Here's how the part is built. I have some questions about the finished solid (model axes, mm). A direction names the side the tool comes from. Round coordinates to 2 decimals unless told otherwise and drop trailing zeros. Write each loop counter-clockwise with the first axis right and the second up, starting at its lowest first coordinate (ties: lowest second). Pieces come first, ordered by that corner, then holes. Notation, with made-up numbers: (49, 35.5) -> (53, 35.5) arc R22 cw to (53, 56.5) -> close; hole circle Ø8 at (25.5, 5.25). An arc over 180 degrees is marked (long way). Answer in a Markdown table with one row per item.
from build123d import *

# Parameters (mm, degrees)
EXTRUDE_1_DEPTH                = 50
SPLIT_BODIES_1_SURFACE_1_BACK  = 226.829
SPLIT_BODIES_1_SURFACE_1_DEPTH = 453.658
SPLIT_BODIES_1_SURFACE_2_BACK  = 226.829
SPLIT_BODIES_1_SURFACE_2_DEPTH = 453.658


with BuildPart() as part:
    # 草图2 → 凸台-拉伸1 (new, symmetric)
    with BuildSketch(Plane.XY):
        with BuildLine():
            Line((120.381757685, 47.561632043), (136.603924057, 47.561632043))
            Line((136.603924057, 47.561632043), (146.850265064, 88.947420909))
            ThreePointArc((146.850265064, 88.947420909), (104.62030332, 85.070472378), (109.988846824, 127.136838271))
            Line((109.988846824, 127.136838271), (88.280849451, 128.197534042))
            ThreePointArc((88.280849451, 128.197534042), (80.571822415, 123.964886157), (80.863683371, 115.175163571))
            ThreePointArc((80.863683371, 115.175163571), (88.300101913, 100.587398022), (92.288223879, 84.706651578))
            Line((92.288223879, 84.706651578), (52.259104564, 84.706651578))
            Line((52.259104564, 84.706651578), (52.259104564, 37.347972633))
            Line((52.259104564, 37.347972633), (26.12059868, 28.530814049))
            Line((26.12059868, 28.530814049), (0, 28.530814049))
            Line((0, 28.530814049), (0, 0))
            Line((0, 0), (140.98, 0))
            Line((140.98, 0), (131.928221984, 26.834036233))
            Line((131.928221984, 26.834036233), (115.249995775, 26.834036233))
            Line((115.249995775, 26.834036233), (120.381757685, 47.561632043))
        make_face()
        with BuildLine():
            ThreePointArc((109.988846824, 127.136838271), (104.62030332, 85.070472378), (146.850265064, 88.947420909))
            Line((146.850265064, 88.947420909), (151.231226865, 106.642475172))
            ThreePointArc((151.231226865, 106.642475172), (147.884639105, 117.258207331), (140.564064785, 125.64287253))
            Line((140.564064785, 125.64287253), (109.988846824, 127.136838271))
        make_face()
        with BuildLine():
            ThreePointArc((140.564064785, 125.64287253), (125.506724817, 131.102497099), (109.988846824, 127.136838271))
            Line((109.988846824, 127.136838271), (140.564064785, 125.64287253))
        make_face()
        with BuildLine():
            ThreePointArc((140.564064785, 125.64287253), (147.884639105, 117.258207331), (151.231226865, 106.642475172))
            Line((151.231226865, 106.642475172), (154.115877694, 118.293810031))
            ThreePointArc((154.115877694, 118.293810031), (153.172952645, 122.982290954), (148.95330104, 125.232957822))
            Line((148.95330104, 125.232957822), (140.564064785, 125.64287253))
        make_face()
    extrude(amount=EXTRUDE_1_DEPTH, both=True)


with BuildPart() as body_2:
    # Split Bodies 1: the piece behind the surface
    add(part.part)
    # Split Bodies 1 surface: a surface, the sketch's curves swept straight by 453.658 mm
    with BuildLine(Plane.XY.offset(50).offset(-SPLIT_BODIES_1_SURFACE_1_BACK), mode=Mode.PRIVATE) as split_bodies_1_surface_1_path:
        Line((120.381757685, 47.561632043), (52.259104564, 47.561632043))
    split_bodies_1_surface_1 = Shell.extrude(split_bodies_1_surface_1_path.wire(), (0 * SPLIT_BODIES_1_SURFACE_1_DEPTH, 0 * SPLIT_BODIES_1_SURFACE_1_DEPTH, 1 * SPLIT_BODIES_1_SURFACE_1_DEPTH))
    split(bisect_by=split_bodies_1_surface_1, keep=Keep.BOTTOM)


with BuildPart() as part_1:
    add(part.part)

    # Split Bodies 1: split by a surface, the side it looks to stays
    # Split Bodies 1 surface: a surface, the sketch's curves swept straight by 453.658 mm
    with BuildLine(Plane.XY.offset(50).offset(-SPLIT_BODIES_1_SURFACE_2_BACK), mode=Mode.PRIVATE) as split_bodies_1_surface_2_path:
        Line((120.381757685, 47.561632043), (52.259104564, 47.561632043))
    split_bodies_1_surface_2 = Shell.extrude(split_bodies_1_surface_2_path.wire(), (0 * SPLIT_BODIES_1_SURFACE_2_DEPTH, 0 * SPLIT_BODIES_1_SURFACE_2_DEPTH, 1 * SPLIT_BODIES_1_SURFACE_2_DEPTH))
    split(bisect_by=split_bodies_1_surface_2, keep=Keep.TOP)


solid = body_2.part
1) I want a section at C-C, the plane y = 95.5. List the corners of the cut face in (x, z) for me, and give its area (3 significant figures).
Response:
| item | result |
|---|---|
| outline | (90, -50) -> (148.47, -50) -> (148.47, 50) -> (90, 50) -> close |
| area | 5,850 mm^2 |
2) I want a section at B-B, the plane x = 65.5. List the corners of the cut face in (y, z) for me.
Response:
| item | result |
|---|---|
| outline | (47.56, -50) -> (84.71, -50) -> (84.71, 50) -> (47.56, 50) -> close |
3) For pin 1 (2 mm diameter, centred on x = 78, z = -33.5, fed in from +Y); pin 2 (8 mm diameter, centred on y = 87, z = 25, fed in from -X); pin 3 (1 mm diameter, centred on x = 107, z = 22, fed in from +Y); pin 4 (5 mm diameter, centred on x = 140.5, z = -22, fed in from +Y), each with a flat end and sliding along its axis, tell me the tip position at first contact or that it passes through.
Response:
| item | result |
|---|---|
| pin 1 | stops at y = 84.71 |
| pin 2 | stops at x = 52.26 |
| pin 3 | stops at y = 127.31 |
| pin 4 | stops at y = 127.36 |
4) We'd pull the mould along Y, two halves only. Please class faces 3 (the face through (99.29, 127.66, 0.7)), 4 (the face through (52.259, 66, 1)), 5 (the face through (88.22, 100.8, 0.7)), 6 (the face through (94, 47.562, 1)): +Y half, -Y half, draft (parallel to the pull), parting line (faces both ways), or undercut.
Response:
| item | result |
|---|---|
| face 3 | +Y half |
| face 4 | draft |
| face 5 | undercut |
| face 6 | -Y half |
5) I want a section at A-A, the plane z = 41.5. List the corners of the cut face in (x, y) for me.
Response:
| item | result |
|---|---|
| outline | (52.26, 47.56) -> (136.6, 47.56) -> (154.12, 118.29) arc R5.6 ccw to (148.95, 125.23) -> (140.56, 125.64) arc R27.18 ccw to (109.99, 127.14) -> (88.28, 128.2) arc R8.4 ccw to (80.86, 115.18) arc R72.8 cw to (92.29, 84.71) -> (52.26, 84.71) -> close |
6) I need wall thicknesses on line 1 (Y direction, x = 68, z = -39); line 2 (Y direction, x = 86.5, z = -29.5); line 3 (Y direction, x = 124.5, z = 7.5). Which ranges of each line are inside material? Lowest first, please. Write a range as [from, to].
Response:
| item | result |
|---|---|
| line 1 | y = [47.56, 84.71] |
| line 2 | y = [47.56, 84.71], [104.95, 128.09] |
| line 3 | y = [47.56, 131.13] |
7) Which directions (+Z, -Z, +X, -X, +Y, -Y) give clear straight access to the entire face, cutting with the end or side of a thin tool? Please do faces 1 (the face through (73, 84.707, 1)), 2 (the face through (144.817, 125.435, 0.7)).
Response:
| item | result |
|---|---|
| face 1 | +Z, -Z, -X |
| face 2 | +Z, -Z, +X, +Y |
